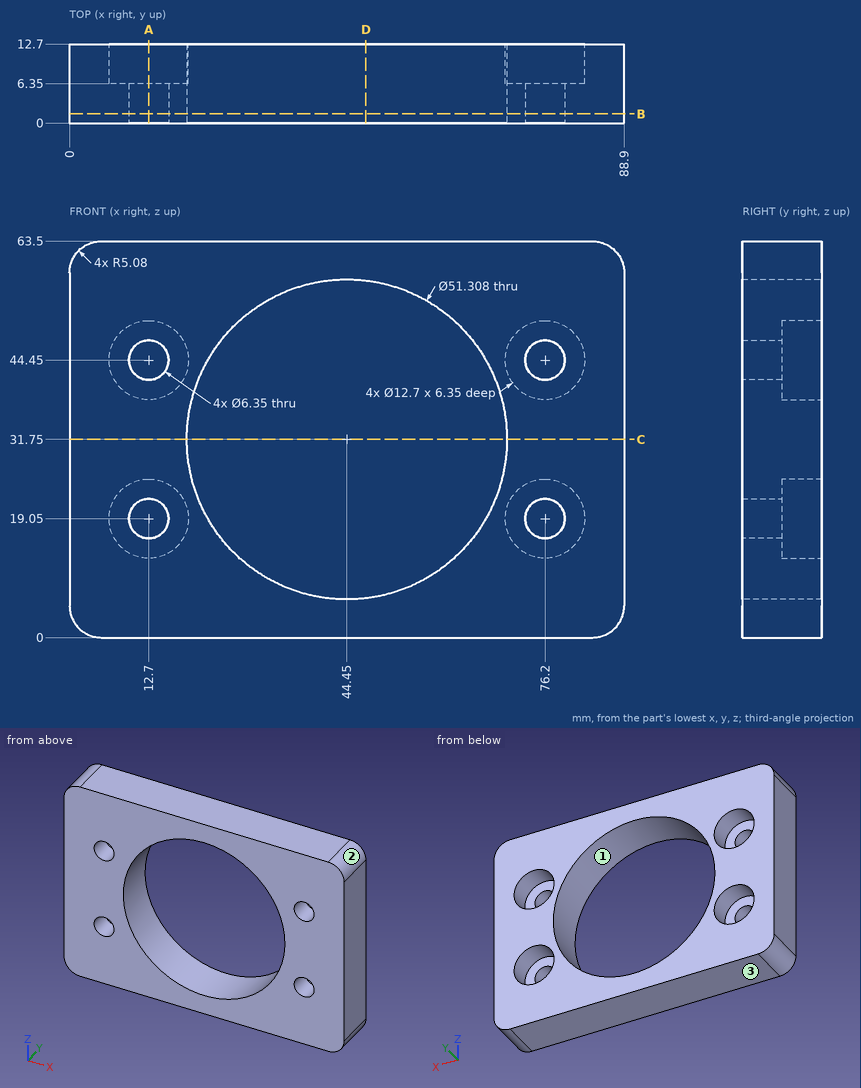
Design review of the part shown in the three views and the two pictorial views. Dimensions are in mm from the part's minimum x, y and z. Coordinates: 2 decimals unless noted, no trailing zeros. Write each loop counter-clockwise with the first axis right and the second up, starting at its lowest first coordinate (ties: lowest second). Pieces come first, ordered by that corner, then holes.
1) We need section D-D on x = 47.5. State the section outline as (y, z) points, then the cut area to 3 significant figures.
2) We need section A-A on x = 12.7. State the section outline as (y, z) points (3 decimals), then the cut area to 3 significant figures.
3) To check wall thickness, follow probe 1 along Z at (x, y) = (76.2, 3.25) (3 decimals); probe 2 along X at (y, z) = (4.25, 44.45) (3 decimals); probe 3 along X at (y, z) = (8.5, 44.45). State the ranges of each line that lie inside material, in increasing order.
4) Clearance check with a flat-ended pin moving along its axis: pin 1 Ø7.5 at (x, z) = (12.7, 19.05) entering from +Y. State where the tip first meets the part, or that it passes through.
5) We need section B-B on y = 1.5. State the section outline as (x, z) points (3 decimals).
6) The part is to be moulded in two halves that separate along X. For the marked faces 1, 2 and 3, say which applies: pulls with the +X half, pulls with the -X half, needs draft (parallel to the pull), parting line crosses it, or undercut.
7) We need section C-C on z = 31.75. State the section outline as (x, y) points, then the cut area to 3 significant figures.
Answer list:
1. outline: (0, 0) - (12.7, 0) - (12.7, 6.28) - (0, 6.28) - close; (0, 57.22) - (12.7, 57.22) - (12.7, 63.5) - (0, 63.5) - close
1. area: 159 mm2
2. outline: (0, 0) - (12.7, 0) - (12.7, 12.7) - (6.35, 12.7) - (6.35, 15.875) - (0, 15.875) - close; (0, 22.225) - (6.35, 22.225) - (6.35, 25.4) - (12.7, 25.4) - (12.7, 38.1) - (6.35, 38.1) - (6.35, 41.275) - (0, 41.275) - close; (0, 47.625) - (6.35, 47.625) - (6.35, 50.8) - (12.7, 50.8) - (12.7, 63.5) - (0, 63.5) - close
2. area: 565 mm2
3. probe 1: z = 0 to 15.875, 22.225 to 41.275, 47.625 to 63.5
3. probe 2: x = 0 to 9.525, 15.875 to 22.16, 66.74 to 73.025, 79.375 to 88.9
3. probe 3: x = 0 to 6.35, 19.05 to 22.16, 66.74 to 69.85, 82.55 to 88.9
4. pin 1: stops at y = 6.35
5. outline: (0, 5.08) arc R5.08 ccw to (5.08, 0) - (83.82, 0) arc R5.08 ccw to (88.9, 5.08) - (88.9, 58.42) arc R5.08 ccw to (83.82, 63.5) - (5.08, 63.5) arc R5.08 ccw to (0, 58.42) - close; hole circle Ø6.35 at (12.7, 19.05); hole circle Ø6.35 at (12.7, 44.45); hole circle Ø51.308 at (44.45, 31.75); hole circle Ø6.35 at (76.2, 19.05); hole circle Ø6.35 at (76.2, 44.45)
6. face 1: undercut
6. face 2: pulls with the +X half
6. face 3: needs draft
7. outline: (0, 0) - (18.8, 0) - (18.8, 12.7) - (0, 12.7) - close; (70.1, 0) - (88.9, 0) - (88.9, 12.7) - (70.1, 12.7) - close
7. area: 477 mm2
